The model under review builds one solid part; all positions refer to its coordinate system, in mm. A direction names the side the tool comes from. Coordinates: 2 decimals unless noted, no trailing zeros. Write each loop counter-clockwise with the first axis right and the second up, starting at its lowest first coordinate (ties: lowest second). Pieces come first, ordered by that corner, then holes. Notation, with made-up numbers: (85, 18.25) - (94, 18.25) arc R29 ccw to (94, 49.25) - close; hole circle Ø1 at (-33.5, -29). An arc over 180 degrees is marked (long way). Return JSON: item names as keys, results as strings. Group by question number.
(1) We need section A-A on z = 3.1. State the section outline as (x, y) points.
(2) We need section B-B on y = 125. State the section outline as (x, z) points.
(3) Tool access review of faces 1 (the face through (-1, 53, 0)), 2 (the face through (-35, 117, 2)), 3 (the face through (35, 117, 2)): name each direction out of +Z, -Z, +X, -X, +Y, -Y from which nothing blocks a thin tool from reaching the whole face with its end or side.
(4) We need section C-C on x = 43. State the section outline as (y, z) points.
(5) To check wall thickness, follow L1, parallel to X at y = 120, z = 4.7; L2, parallel to X at y = 84, z = 4.75; L3, parallel to Y at x = -47.5, z = 3.9. State the ranges of each line that lie inside material, in increasing order. Write a range as from..to.
(6) For pin 1 Ø1 at (x, y) = (-28.5, 42.5) entering from -Z; pin 2 Ø1.5 at (y, z) = (119, 3.5) entering from -X, all flat-tipped, find the tip position at first contact; note any pin that passes through.
```python
from build123d import *

# Parameters (mm, degrees)
F1_DEPTH    = 5
F2_T1_DEPTH = 5


# Not quite as in the source:
# - a fillet or chamfer that OpenCascade refuses, or shapes differently, is made with other operations: its cross-section is extruded or revolved along the edge and cut away or added


with BuildPart() as f1:
    # F0 (on Top) → F1 (new body)
    with BuildSketch(Plane.XY):
        Polygon((35, 135), (-35, 135), (-35, 75), (-55, 75), (-55, 0), (55, 0), (55, 75), (35, 75), align=None)
    extrude(amount=F1_DEPTH)

    # F2: fillet of radius 25 on 2 edges, made by hand

    # F2_s2 → F2_t1 (join)
    with BuildSketch(Plane.XY):
        with BuildLine():
            ThreePointArc((-35, 99.4948974278), (-40.635083269, 83.683509127), (-55, 75))
            Line((-55, 75), (-35, 75))
            Line((-35, 75), (-35, 99.4948974278))
        make_face()
        with BuildLine():
            ThreePointArc((55, 75), (40.635083269, 83.683509127), (35, 99.4948974278))
            Line((35, 99.4948974278), (35, 75))
            Line((35, 75), (55, 75))
        make_face()
    extrude(amount=F2_T1_DEPTH)


solid = f1.part
```
Ans:
{
 "1": {"outline": "(-55, 0) - (55, 0) - (55, 75) arc R25 cw to (35, 99.49) - (35, 135) - (-35, 135) - (-35, 99.49) arc R25 cw to (-55, 75) - close"},
 "2": {"outline": "(-35, 0) - (35, 0) - (35, 5) - (-35, 5) - close"},
 "3": {"face 1": "-Z, +X, -X, +Y, -Y", "face 2": "+Z, -Z, -X, +Y", "face 3": "+Z, -Z, +X, +Y"},
 "4": {"outline": "(0, 0) - (81.16, 0) - (81.16, 5) - (0, 5) - close"},
 "5": {"L1": "-35..35", "L2": "-40.38..40.38", "L3": "0..77.84"},
 "6": {"pin 1": "z = 0", "pin 2": "x = -35"}
}
